Check sheet for the drawn part. Datum: minimum x, y, z corner. Units: mm. Give positions to 0.01 mm unless a question says otherwise; leave off trailing zeros. Order: outer loops, then holes, each group sorted by start corner. A loop starts at its lowest first (then second) coordinate and runs counter-clockwise, first axis right, second up. Notation, with made-up numbers: (-29.75, 44) -> (23.25, 44) arc R29 cw to (23.25, 79) -> close; hole circle Ø10 at (47, -10). An arc over 180 degrees is marked (long way). Answer in a Markdown table with one row per item. Add a question column.
(1) Cross-section at D-D (x = 17.5). Record the cut outline in (y, z), then the cut area to 3 significant figures.
(2) Go/stop test with flat-tipped pins: pin 1 (2 mm diameter, centred on x = 3, y = 35, fed in from -Z); pin 2 (1.5 mm diameter, centred on y = 53.5, z = 1, fed in from -X). Record where each tip stops, or that it passes through.
(3) Cross-section at A-A (y = 34). Record the cut outline in (x, z).
(4) Cross-section at C-C (z = 2). Record the cut outline in (x, y).
(5) Thickness scan on L1, parallel to Y at x = 2, z = 0.5; L2, parallel to X at y = 45, z = 0.2; L3, parallel to Y at x = 7, z = 2.35. Record the ranges inside material, lowest first. Write a range as [from, to].
(6) Cross-section at B-B (x = 9.25). Record the cut outline in (y, z).
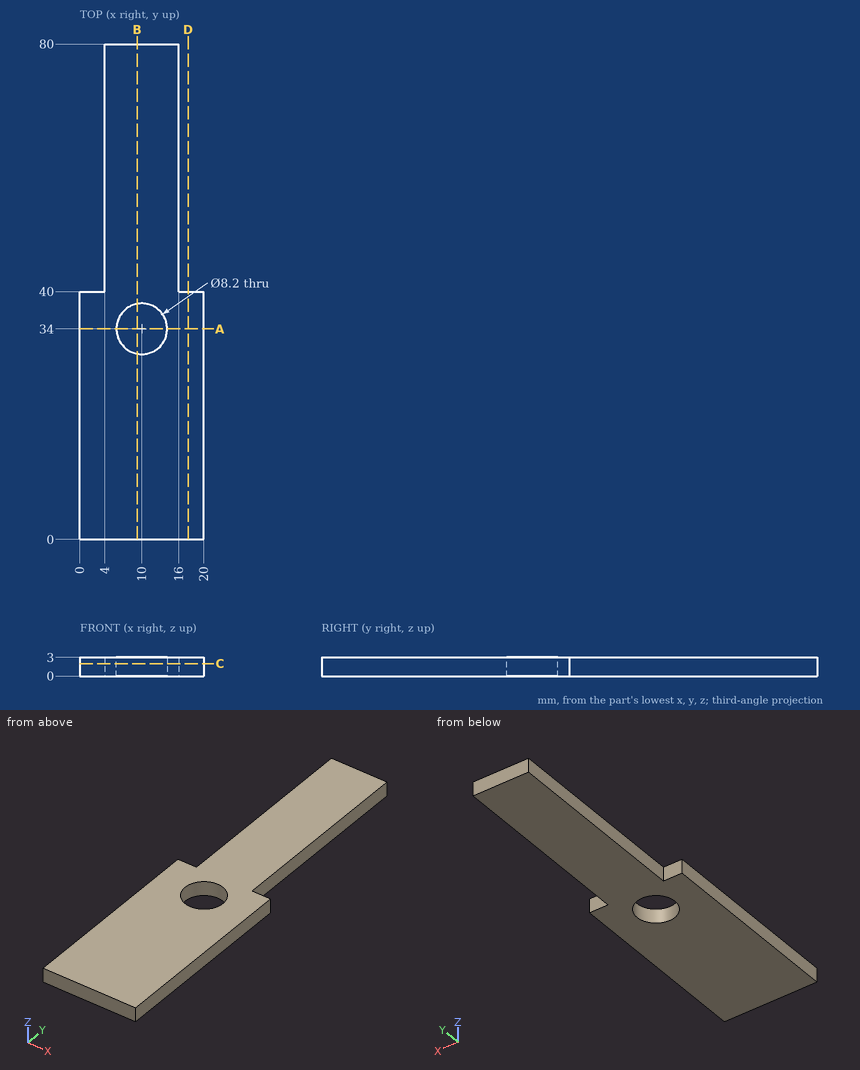
Answer below:
| question | item | result |
|---|---|---|
| 1 | outline | (0, 0) -> (40, 0) -> (40, 3) -> (0, 3) -> close |
| 1 | area | 120 mm² |
| 2 | pin 1 | stops at z = 0 |
| 2 | pin 2 | stops at x = 4 |
| 3 | outline | (0, 0) -> (5.9, 0) -> (5.9, 3) -> (0, 3) -> close; (14.1, 0) -> (20, 0) -> (20, 3) -> (14.1, 3) -> close |
| 4 | outline | (0, 0) -> (20, 0) -> (20, 40) -> (16, 40) -> (16, 80) -> (4, 80) -> (4, 40) -> (0, 40) -> close; hole circle Ø8.2 at (10, 34) |
| 5 | L1 | y = [0, 40] |
| 5 | L2 | x = [4, 16] |
| 5 | L3 | y = [0, 31.21], [36.79, 80] |
| 6 | outline | (0, 0) -> (29.97, 0) -> (29.97, 3) -> (0, 3) -> close; (38.03, 0) -> (80, 0) -> (80, 3) -> (38.03, 3) -> close |
